from build123d import *

# Parameters (mm, degrees)
SKETCH2_R           = 50
BOSS_EXTRUDE1_DEPTH = 80
SKETCH3_W           = 21
SKETCH3_H           = 55
CUT_EXTRUDE2_DEPTH  = 3
SKETCH4_W           = 21
SKETCH4_H           = 40
CUT_EXTRUDE3_DEPTH  = 28
SKETCH5_W           = 21
SKETCH5_H           = 56.862422016
CUT_EXTRUDE4_DEPTH  = 31


with BuildPart() as part:
    # Sketch2 → Boss-Extrude1 (new body)
    with BuildSketch(Plane(origin=(0, 0, 0), x_dir=(1, 0, 0), z_dir=(0, 1, 0))):
        with Locations(Location((0, 0, 0), (0, 0, 270))):
            Circle(SKETCH2_R)
    extrude(amount=BOSS_EXTRUDE1_DEPTH)

    # Sketch3 → Cut-Extrude2 (cut)
    with BuildSketch(Plane(origin=(0, 80, 0), x_dir=(1, 0, 0), z_dir=(0, 1, 0))):
        Rectangle(SKETCH3_W, SKETCH3_H)
    extrude(amount=-CUT_EXTRUDE2_DEPTH, mode=Mode.SUBTRACT)

    # Sketch4 → Cut-Extrude3 (cut)
    with BuildSketch(Plane(origin=(0, 77, 0), x_dir=(1, 0, 0), z_dir=(0, 1, 0))):
        Rectangle(SKETCH4_W, SKETCH4_H)
    extrude(amount=-CUT_EXTRUDE3_DEPTH, mode=Mode.SUBTRACT)

    # Sketch5 → Cut-Extrude4 (cut)
    with BuildSketch(Plane(origin=(0, 80, 0), x_dir=(1, 0, 0), z_dir=(0, 1, 0))):
        with Locations((0, -28.431211008)):
            Rectangle(SKETCH5_W, SKETCH5_H)
    extrude(amount=-CUT_EXTRUDE4_DEPTH, mode=Mode.SUBTRACT)


solid = part.part
Could you check a few things on this model? Use its own coordinates, in mm. A direction names the side the tool comes from. Round coordinates to 2 decimals unless told otherwise and drop trailing zeros. Order: outer loops, then holes, each group sorted by start corner. A loop starts at its lowest first (then second) coordinate and runs counter-clockwise, first axis right, second up.
(1) Imagine slicing it at A-A (z = 0). Write out the boundary of the cut face in (x, y), plus the area to 3 significant figures.
Response values:
outline: (-50, 0) - (50, 0) - (50, 80) - (10.5, 80) - (10.5, 49) - (-10.5, 49) - (-10.5, 80) - (-50, 80) - close
area: 7,350 mm2
(2) If we mould it in two halves opening along X, with no side actions, what happens to faces 1 (the flat face through (10.5, 65, 11)), 2 (the cylindrical face through (15.02, 39.44, 47.69)), 3 (the flat face through (1, 0, -1)), 4 (the flat face through (0, 49, 15))? For each: released by +X, released by -X, zero draft, split by the parting line, or undercut.
Response values:
face 1: undercut
face 2: split by the parting line
face 3: zero draft
face 4: undercut
(3) Imagine slicing it at B-B (x = 0). Write out the boundary of the cut face in (y, z).
Response values:
outline: (0, -50) - (80, -50) - (80, -27.5) - (77, -27.5) - (77, -20) - (49, -20) - (49, 50) - (0, 50) - close
(4) Please list where these lines run through material, in increasing order: line 1 along X through (y, z) = (51, -8.5); line 2 along Y through (x, z) = (-10, 8.5); line 3 along Z through (x, y) = (0.5, 56).
Response values:
line 1: x = -49.27 to -10.5, 10.5 to 49.27
line 2: y = 0 to 49
line 3: z = -50 to -20
(5) Imagine slicing it at D-D (y = 11.5). Write out the boundary of the cut face in (x, z).
Response values:
outline: circle Ø100 at (0, 0)
(6) Imagine slicing it at C-C (y = 61.5). Write out the boundary of the cut face in (x, z).
Response values:
outline: (-10.5, -20) - (-10.5, 48.89) arc R50 ccw (long way) to (10.5, 48.89) - (10.5, -20) - close
(7) I'm going to push flat-ended pins straight in: pin 1 (4 mm diameter, centred on x = -30, y = 65.5, fed in from +Z); pin 2 (25 mm diameter, centred on y = 58.5, z = 15, fed in from -X); pin 3 (10.5 mm diameter, centred on x = -4, z = 12, fed in from +Y). Where does each tip first touch, or does it pass through?
Response values:
pin 1: stops at z = 41.42
pin 2: stops at x = -49.94
pin 3: stops at y = 49
(8) Which directions (+Z, -Z, +X, -X, +Y, -Y) give clear straight access to the entire face, cutting with the end or side of a thin tool? Please do faces 5 (the flat face through (-10.5, 65, 11)), 6 (the flat face through (12, 80, -1)).
Response values:
face 5: +Z, +Y
face 6: +Z, -Z, +X, -X, +Y
